Source: CAD feature listing. Evaluate the final solid. Frame: model axes, mm. Face numbers are marked on the shaded views. Give positions to 0.01 mm unless a question says otherwise; leave off trailing zeros. Order: outer loops, then holes, each group sorted by start corner. A loop starts at its lowest first (then second) coordinate and runs counter-clockwise, first axis right, second up.
1) Section C-C, the plane y = 27.5. Return loops of the section in (x, z), plus the area to 3 significant figures.
2) First-contact query: P1, Ø7, axis at x = 2, z = 10, coming from the +Y side; P2, Ø2, axis at x = -52, y = -28, coming from the -Z side. Flat tips, straight axial feed; report the tip coordinate or a pass-through.
3) Section A-A, the plane x = 3. Return loops of the section in (y, z), plus the area to 3 significant figures.
4) Material intervals for line 1 (X direction, y = -40, z = 1.5); line 2 (Z direction, x = -11.5, y = -25.5); line 3 (Y direction, x = -78, z = 11), sorted ascending.
5) Section B-B, the plane z = 5.25. Return loops of the section in (x, y), plus the area to 3 significant figures.
6) Draft query along X for the marked faces 1, 2, 3 and 4. Return one class per face: released by +X, released by -X, zero draft, split by the parting line, or undercut.
```python
from build123d import *

# Parameters (mm, degrees)
F1_DEPTH = 15.9
F2_DEPTH = 13.9
F3_DEPTH = 1


with BuildPart() as f1:
    # F0 (on Top) → F1 (new body)
    with BuildSketch(Plane.XY):
        Polygon((-84.823024, -30.93472), (-84.823024, 44.51528), (-86.823024, 44.51528), (-86.823024, -48.93472), (72.176976, -48.93472), (72.176976, 44.51528), (70.176976, 44.51528), (70.176976, -30.93472), (70.176976, -46.93472), (58.176976, -46.93472), (-72.823024, -46.93472), (-84.823024, -46.93472), align=None)
        Polygon((-72.823024, -46.93472), (-84.823024, -30.93472), (-84.823024, -46.93472), align=None)
        Polygon((70.176976, -46.93472), (70.176976, -30.93472), (58.176976, -46.93472), align=None)
        Polygon((70.176976, 44.51528), (-84.823024, 44.51528), (-84.823024, -30.93472), (-72.823024, -46.93472), (58.176976, -46.93472), (70.176976, -30.93472), align=None)
    extrude(amount=F1_DEPTH)

    # F0 (on Top) → F2 (cut)
    with BuildSketch(Plane.XY):
        Polygon((-72.823024, -46.93472), (-84.823024, -30.93472), (-84.823024, -46.93472), align=None)
        Polygon((70.176976, 44.51528), (-84.823024, 44.51528), (-84.823024, -30.93472), (-72.823024, -46.93472), (58.176976, -46.93472), (70.176976, -30.93472), align=None)
        Polygon((70.176976, -46.93472), (70.176976, -30.93472), (58.176976, -46.93472), align=None)
    extrude(amount=F2_DEPTH, mode=Mode.SUBTRACT)

    # F0 (on Top) → F3 (join)
    with BuildSketch(Plane.XY):
        Polygon((-72.823024, -46.93472), (-84.823024, -30.93472), (-84.823024, -46.93472), align=None)
        Polygon((70.176976, -46.93472), (70.176976, -30.93472), (58.176976, -46.93472), align=None)
    extrude(amount=F3_DEPTH)


solid = f1.part
```
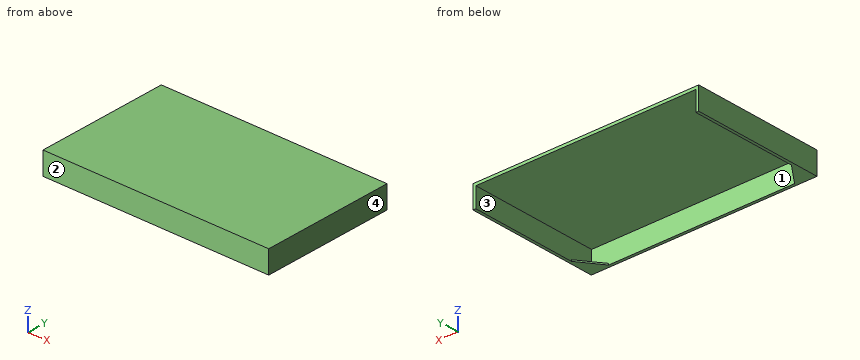
From the geometry:
1. outline: (-86.82, 0) - (-84.82, 0) - (-84.82, 13.9) - (70.18, 13.9) - (70.18, 0) - (72.18, 0) - (72.18, 15.9) - (-86.82, 15.9) - close
1. area: 374 mm2
2. P1: stops at y = -46.93
2. P2: stops at z = 13.9
3. outline: (-48.93, 0) - (-46.93, 0) - (-46.93, 13.9) - (44.52, 13.9) - (44.52, 15.9) - (-48.93, 15.9) - close
3. area: 215 mm2
4. line 1: x = -86.82 to -84.82, 70.18 to 72.18
4. line 2: z = 13.9 to 15.9
4. line 3: y = -48.93 to -46.93
5. outline: (-86.82, -48.93) - (72.18, -48.93) - (72.18, 44.52) - (70.18, 44.52) - (70.18, -46.93) - (-84.82, -46.93) - (-84.82, 44.52) - (-86.82, 44.52) - close
5. area: 684 mm2
6. face 1: undercut
6. face 2: zero draft
6. face 3: undercut
6. face 4: released by +X
